Geometry: see drawing. Coordinates: mm, zero at the bounding-box minimum. Give positions to 0.01 mm unless a question says otherwise; leave off trailing zeros. Loops run counter-clockwise (first coordinate to the right, second up) from the corner with the lowest first, then second, coordinate; pieces in that order, holes last. Notation, with made-up numbers: M 35.5,-19 L 92.5,-19 A20 ccw 92.5,-11 Z; hole C -4,19.5 d5. An arc over 180 degrees is marked long. Use a Markdown table: item, result. Add a question column.
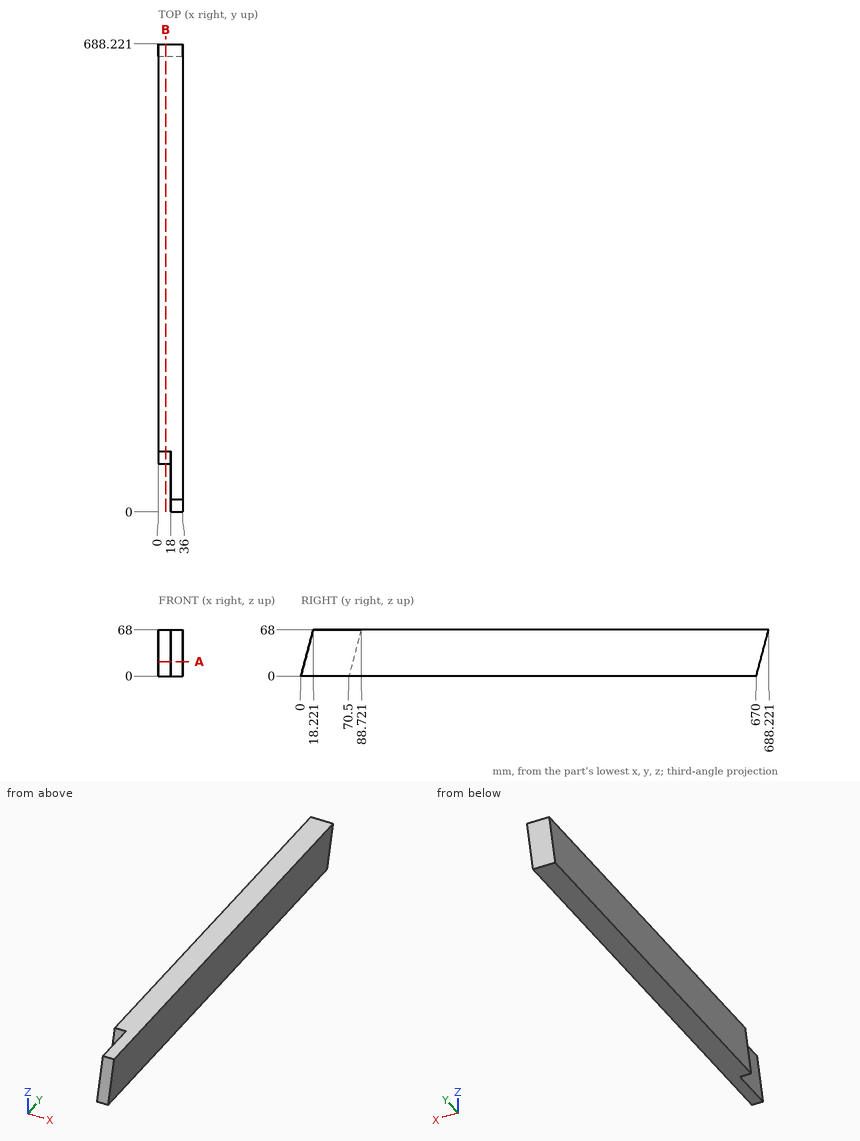
1) Section query A-A, the plane z = 21. Return the cut outline in (x, y).
2) Ray query, line 1 (Y direction, x = 2, z = 7.5); line 2 (Y direction, x = 12, z = 53). Return the intervals inside material, ascending. Write a range as [from, to].
3) Contact query for flat-ended pins moving along their axis: P1, Ø5, axis at x = 30.5, z = 8.5, coming from the +Y side; P2, Ø1.5, axis at x = 11.5, z = 53.5, coming from the -Y side (1 decimal); P3, Ø5, axis at y = 351, z = 33, coming from the -X side; P4, Ø12, axis at x = 25, z = 28.5, coming from the +Y side (1 decimal). Output: stop coordinate, or through.
4) Section query B-B, the plane x = 10.5. Return the cut outline in (y, z).
Entries:
| question | item | result |
|---|---|---|
| 1 | outline | M 0,76.13 L 18,76.13 L 18,5.63 L 36,5.63 L 36,675.63 L 0,675.63 Z |
| 2 | line 1 | y = [72.51, 672.01] |
| 2 | line 2 | y = [84.7, 684.2] |
| 3 | P1 | stops at y = 672.95 |
| 3 | P2 | stops at y = 84.6 |
| 3 | P3 | stops at x = 0 |
| 3 | P4 | stops at y = 679.2 |
| 4 | outline | M 70.5,0 L 670,0 L 688.22,68 L 88.72,68 Z |
